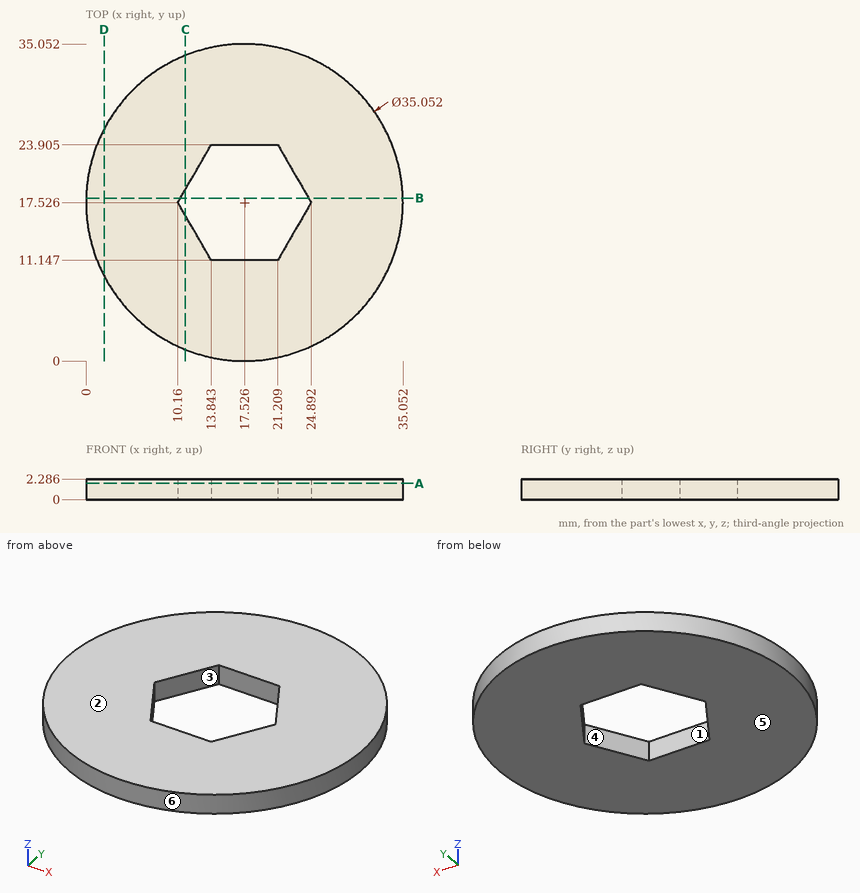
Design review of the part shown in the three views and the two pictorial views. Dimensions are in mm from the part's minimum x, y and z. A direction names the side the tool comes from. Round coordinates to 2 decimals unless told otherwise and drop trailing zeros. Loops run counter-clockwise (first coordinate to the right, second up) from the corner with the lowest first, then second, coordinate; pieces in that order, holes last.
(1) Mouldability with a two-part tool opening along Y and no side actions: class the marked faces 3, 4, 5 and 6 as released by +Y, released by -Y, zero draft, split by the parting line, or undercut.
Returned:
face 3: undercut
face 4: undercut
face 5: zero draft
face 6: split by the parting line
(2) Tool access review of the marked faces 1 and 2: name each direction out of +Z, -Z, +X, -X, +Y, -Y from which nothing blocks a thin tool from reaching the whole face with its end or side.
Returned:
face 1: +Z, -Z
face 2: +Z, +X, -X, +Y, -Y
(3) Wall thickness on line 1 along Y through (x, z) = (18, 1.05) (1 decimal); line 2 along X through (y, z) = (13.5, 2.05) (1 decimal); line 3 along X through (y, z) = (20, 1.5) (1 decimal): over which ranges is each line inside the solid? List them lowest first.
Returned:
line 1: y = 0 to 11.1, 23.9 to 35
line 2: x = 0.5 to 12.5, 22.6 to 34.6
line 3: x = 0.2 to 11.6, 23.5 to 34.9
(4) We need section A-A (z = 1.8). Give the boundary of the cut face in (x, y) (3 decimals), plus the area to 3 significant figures.
Returned:
outline: circle Ø35.052 at (17.526, 17.526); hole (10.16, 17.526) - (13.843, 11.147) - (21.209, 11.147) - (24.892, 17.526) - (21.209, 23.905) - (13.843, 23.905) - close
area: 824 mm2
(5) We need section C-C (x = 11). Give the boundary of the cut face in (y, z), plus the area to 3 significant figures.
Returned:
outline: (1.26, 0) - (16.07, 0) - (16.07, 2.29) - (1.26, 2.29) - close; (18.98, 0) - (33.79, 0) - (33.79, 2.29) - (18.98, 2.29) - close
area: 67.7 mm2
(6) We need section D-D (x = 2). Give the boundary of the cut face in (y, z).
Returned:
outline: (9.4, 0) - (25.66, 0) - (25.66, 2.29) - (9.4, 2.29) - close
(7) We need section B-B (y = 18). Give the boundary of the cut face in (x, z), plus the area to 3 significant figures.
Returned:
outline: (0.01, 0) - (10.43, 0) - (10.43, 2.29) - (0.01, 2.29) - close; (24.62, 0) - (35.05, 0) - (35.05, 2.29) - (24.62, 2.29) - close
area: 47.7 mm2
